Geometry check sheet. Reference: drawing and pictorial views, mm from the part's lowest x, y, z. Give positions to 0.01 mm unless a question says otherwise; leave off trailing zeros. Loops run counter-clockwise (first coordinate to the right, second up) from the corner with the lowest first, then second, coordinate; pieces in that order, holes last. Notation, with made-up numbers: (89.5, -2) -> (106.5, -2) arc R33 ccw to (106.5, 30) -> close; hole circle Ø10 at (18, 87.5). An arc over 180 degrees is marked (long way). Write each question's results on one line, items separated by ' | '. Start each with the question number.
1. Gauge pin test, flat end, axial feed: pin 1 Ø2 at (x, y) = (5, 125) entering from -Z. Record the tip position at first contact, or that the pin passes through.
2. Cross-section at A-A on y = 5. Record the boundary of the cut face in (x, z).
3. Material ranges on L1, parallel to Y at x = 5, z = 2.9; L2, parallel to X at y = 125, z = 1.6; L3, parallel to Y at x = 69, z = 4.45, recorded low to high. Write a range as from..to.
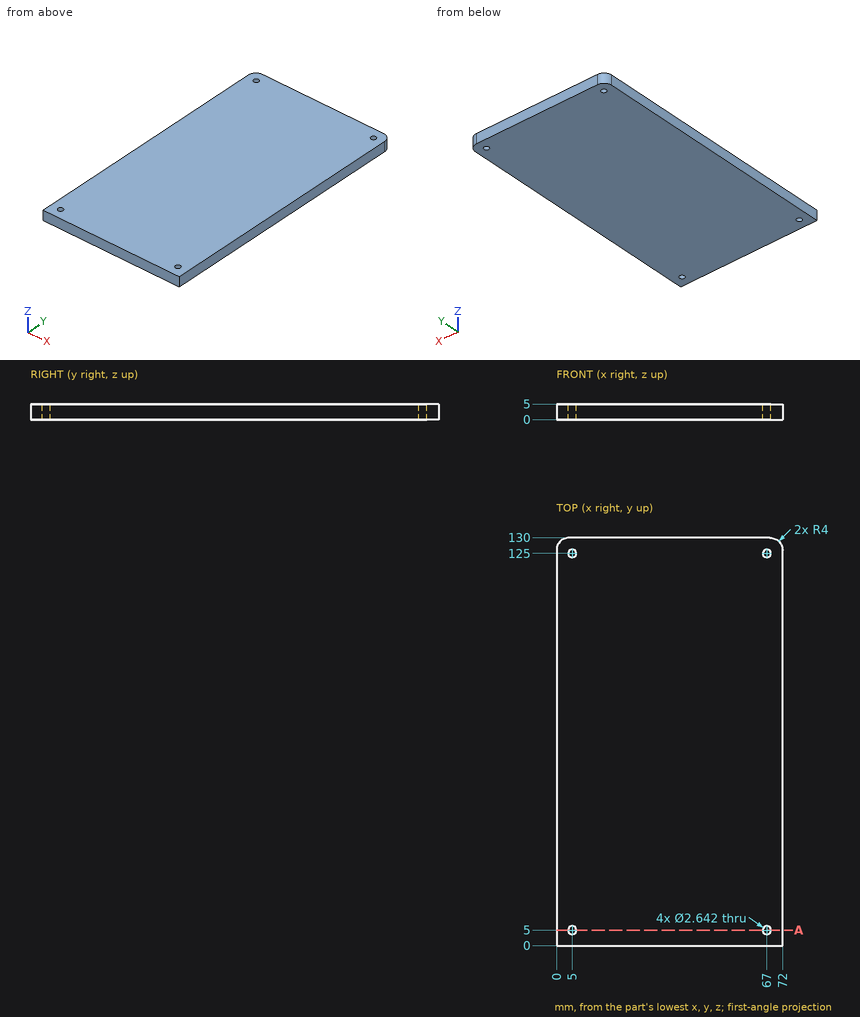
Geometry says:
1) pin 1: through
2) outline: (0, 0) -> (3.68, 0) -> (3.68, 5) -> (0, 5) -> close; (6.32, 0) -> (65.68, 0) -> (65.68, 5) -> (6.32, 5) -> close; (68.32, 0) -> (72, 0) -> (72, 5) -> (68.32, 5) -> close
3) L1: 0..3.68, 6.32..123.68, 126.32..130 | L2: 0..3.68, 6.32..65.68, 68.32..72 | L3: 0..129.87
